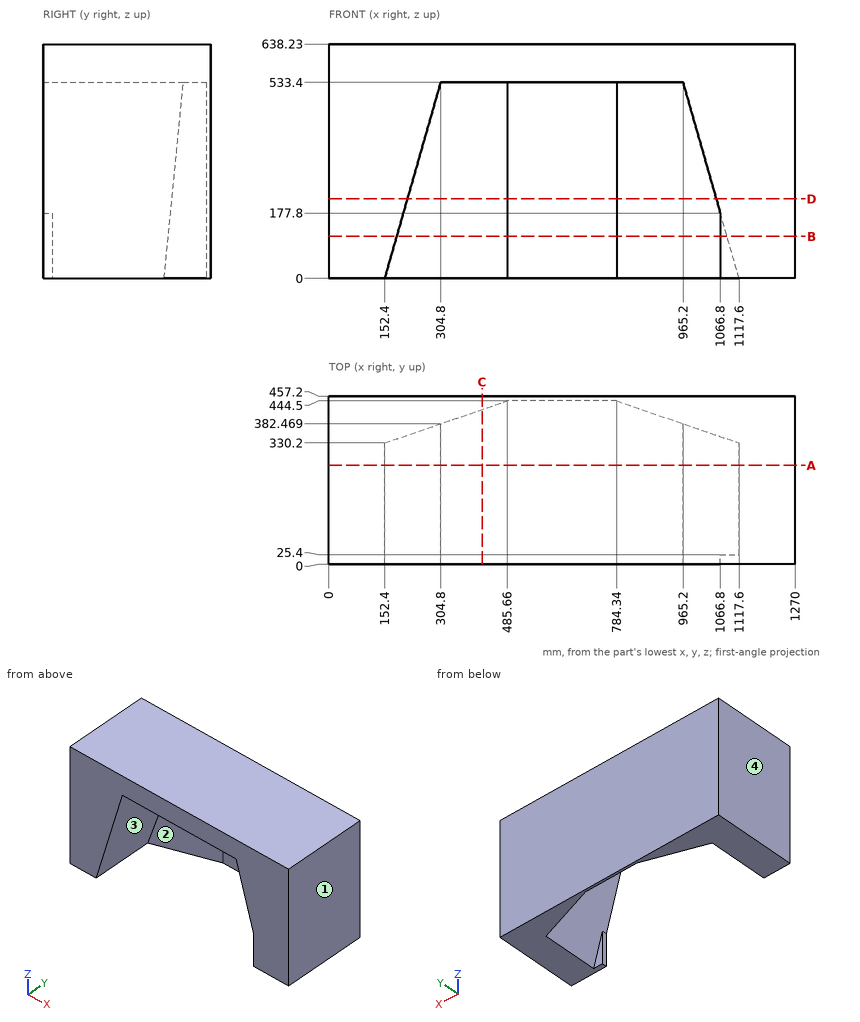
Geometry check sheet. Reference: drawing and pictorial views, mm from the part's lowest x, y, z. Coordinates: 2 decimals unless noted, no trailing zeros. Write each loop counter-clockwise with the first axis right and the second up, starting at its lowest first coordinate (ties: lowest second). Pieces come first, ordered by that corner, then holes.
Item 1: Cross-section at A-A on y = 269. Record the boundary of the cut face in (x, z).
Numbers:
outline: (0, 0) - (152.4, 0) - (304.8, 533.4) - (965.2, 533.4) - (1117.6, 0) - (1270, 0) - (1270, 638.23) - (0, 638.23) - close
Item 2: Cross-section at D-D on z = 216. Record the boundary of the cut face in (x, y) (1 decimal).
Numbers:
outline: (0, 0) - (214.1, 0) - (214.1, 351.4) - (485.7, 444.5) - (784.3, 444.5) - (1055.9, 351.4) - (1055.9, 0) - (1270, 0) - (1270, 457.2) - (0, 457.2) - close
Item 3: Depth check by flat-ended pin: pin 1 Ø10 at (x, z) = (310.5, 111) entering from -Y; pin 2 Ø8 at (x, y) = (715, 228) entering from -Z. Enter the tip coordinate at first touch or a pass-through.
Numbers:
pin 1: stops at y = 382.71
pin 2: stops at z = 533.4
Item 4: Scan lines: probe 1 along X at (y, z) = (131.5, 36) (1 decimal); probe 2 along Z at (x, y) = (714.5, 173.5); probe 3 along X at (y, z) = (39.5, 28). Record each from-to range of solid material in increasing order.
Numbers:
probe 1: x = 0 to 162.7, 1107.3 to 1270
probe 2: z = 533.4 to 638.23
probe 3: x = 0 to 160.4, 1109.6 to 1270
Item 5: Mould release check, pull along X, two halves, no side actions. Record for the marked faces 1, 2, 3 and 4: released by +X, released by -X, zero draft, split by the parting line, or undercut.
Numbers:
face 1: released by +X
face 2: undercut
face 3: undercut
face 4: released by -X
Item 6: Cross-section at B-B on z = 114. Record the boundary of the cut face in (x, y).
Numbers:
outline: (0, 0) - (184.97, 0) - (184.97, 341.37) - (485.66, 444.5) - (784.34, 444.5) - (1085.03, 341.37) - (1085.03, 25.4) - (1066.8, 25.4) - (1066.8, 0) - (1270, 0) - (1270, 457.2) - (0, 457.2) - close
Item 7: Cross-section at C-C on x = 417.5. Record the boundary of the cut face in (y, z), then the cut area to 3 significant figures.
Numbers:
outline: (0, 533.4) - (421.12, 533.4) - (421.12, 0) - (457.2, 0) - (457.2, 638.23) - (0, 638.23) - close
area: 67,200 mm2
